Build history of the part. All positions in model axes, mm. Give positions to 0.01 mm unless a question says otherwise; leave off trailing zeros. Order: outer loops, then holes, each group sorted by start corner. A loop starts at its lowest first (then second) coordinate and runs counter-clockwise, first axis right, second up. Notation, with made-up numbers: (42, -31.5) - (60, -31.5) arc R13 cw to (60, -9.5) - close; hole circle Ø6 at (4, -28). An arc over 180 degrees is marked (long way). Use a Markdown table: item, result.
from build123d import *

# Parameters (mm, degrees)
SKETCH1_W           = 63.5
SKETCH1_H           = 88.9
SKETCH1_R           = 3.429
BOSS_EXTRUDE1_DEPTH = 6
FILLET1_R           = 10.16
SKETCH2_R           = 2.54
CUT_EXTRUDE1_DEPTH  = 110.414167273


with BuildPart() as part:
    # Sketch1 → Boss-Extrude1 (new body)
    with BuildSketch(Plane(origin=(0, 0, 0), x_dir=(1, 0, 0), z_dir=(0, 1, 0))):
        with Locations((31.75, 44.45)):
            Rectangle(SKETCH1_W, SKETCH1_H)
        with Locations(Location((17.78, 73.025, 0), (0, 0, 270))):
            Circle(SKETCH1_R, mode=Mode.SUBTRACT)
        with Locations(Location((45.72, 15.875, 0), (0, 0, 270))):
            Circle(SKETCH1_R, mode=Mode.SUBTRACT)
        with Locations(Location((17.78, 15.875, 0), (0, 0, 90))):
            Circle(SKETCH1_R, mode=Mode.SUBTRACT)
        with Locations(Location((45.72, 73.025, 0), (0, 0, 90))):
            Circle(SKETCH1_R, mode=Mode.SUBTRACT)
    extrude(amount=BOSS_EXTRUDE1_DEPTH)

    # Fillet1
    fillet1_edges = [part.edges().sort_by_distance(p)[0] for p in [
        (0, 3, -88.9),
        (63.5, 3, -88.9),
        (63.5, 3, 0),
        (0, 3, 0),
    ]]
    fillet(fillet1_edges, radius=FILLET1_R)

    # Sketch2 → Cut-Extrude1 (cut, through all)
    with BuildSketch(Plane(origin=(0, 6, 0), x_dir=(1, 0, 0), z_dir=(0, 1, 0))):
        with Locations(Location((6.35, 31.75, 0), (0, 0, 270))):
            Circle(SKETCH2_R)
        with Locations(Location((6.35, 44.45, 0), (0, 0, 270))):
            Circle(SKETCH2_R)
        with Locations(Location((6.35, 57.15, 0), (0, 0, 270))):
            Circle(SKETCH2_R)
        with Locations(Location((19.05, 57.15, 0), (0, 0, 270))):
            Circle(SKETCH2_R)
        with Locations(Location((19.05, 44.45, 0), (0, 0, 270))):
            Circle(SKETCH2_R)
        with Locations(Location((19.05, 31.75, 0), (0, 0, 270))):
            Circle(SKETCH2_R)
        with Locations(Location((31.75, 31.75, 0), (0, 0, 270))):
            Circle(SKETCH2_R)
        with Locations(Location((31.75, 44.45, 0), (0, 0, 270))):
            Circle(SKETCH2_R)
        with Locations(Location((31.75, 57.15, 0), (0, 0, 270))):
            Circle(SKETCH2_R)
        with Locations(Location((44.45, 57.15, 0), (0, 0, 270))):
            Circle(SKETCH2_R)
        with Locations(Location((44.45, 44.45, 0), (0, 0, 270))):
            Circle(SKETCH2_R)
        with Locations(Location((57.15, 44.45, 0), (0, 0, 270))):
            Circle(SKETCH2_R)
        with Locations(Location((57.15, 31.75, 0), (0, 0, 270))):
            Circle(SKETCH2_R)
        with Locations(Location((44.45, 31.75, 0), (0, 0, 270))):
            Circle(SKETCH2_R)
        with Locations(Location((57.15, 57.15, 0), (0, 0, 270))):
            Circle(SKETCH2_R)
    extrude(amount=-CUT_EXTRUDE1_DEPTH, mode=Mode.SUBTRACT)


solid = part.part
1) Two-plate mould, pull along X, no slides. Class faces 1 (the flat face through (63.5, 3, -44)), 2 (the cylindrical face through (17.63, 2.96, -12.45)), 3 (the cylindrical face through (2.897, 3.042, -3.055)): +X half, -X half, draft (parallel to the pull), parting line (faces both ways), or undercut.
Computed:
| item | result |
|---|---|
| face 1 | +X half |
| face 2 | undercut |
| face 3 | -X half |
2) Slice it at B-B (y = 2.6). State how many separate pieces and enclosed holes the cut face has, and give its area (3 significant figures).
Computed:
| item | result |
|---|---|
| separate pieces | 1 |
| enclosed holes | 19 |
| area | 5,100 mm² |
3) Slice it at C-C (z = -31.75). Write the cut outline in (x, y).
Computed:
| item | result |
|---|---|
| outline | (0, 0) - (3.81, 0) - (3.81, 6) - (0, 6) - close; (8.89, 0) - (16.51, 0) - (16.51, 6) - (8.89, 6) - close; (21.59, 0) - (29.21, 0) - (29.21, 6) - (21.59, 6) - close; (34.29, 0) - (41.91, 0) - (41.91, 6) - (34.29, 6) - close; (46.99, 0) - (54.61, 0) - (54.61, 6) - (46.99, 6) - close; (59.69, 0) - (63.5, 0) - (63.5, 6) - (59.69, 6) - close |
4) Slice it at A-A (x = 31.75). Write the cut outline in (y, z).
Computed:
| item | result |
|---|---|
| outline | (0, -88.9) - (6, -88.9) - (6, -59.69) - (0, -59.69) - close; (0, -54.61) - (6, -54.61) - (6, -46.99) - (0, -46.99) - close; (0, -41.91) - (6, -41.91) - (6, -34.29) - (0, -34.29) - close; (0, -29.21) - (6, -29.21) - (6, 0) - (0, 0) - close |
5) Slice it at D-D (x = 45.72). Write the cut outline in (y, z).
Computed:
| item | result |
|---|---|
| outline | (0, -88.9) - (6, -88.9) - (6, -76.45) - (0, -76.45) - close; (0, -69.6) - (6, -69.6) - (6, -59.35) - (0, -59.35) - close; (0, -54.95) - (6, -54.95) - (6, -46.65) - (0, -46.65) - close; (0, -42.25) - (6, -42.25) - (6, -33.95) - (0, -33.95) - close; (0, -29.55) - (6, -29.55) - (6, -19.3) - (0, -19.3) - close; (0, -12.45) - (6, -12.45) - (6, 0) - (0, 0) - close |
6) Wall check: line 1 (X direction, y = 4.45, z = -16); line 2 (X direction, y = 1.6, z = -57.15); line 3 (Z direction, x = 55, y = 4.5). Give the ranges that are in metal, low to high. Write a range as from..to.
Computed:
| item | result |
|---|---|
| line 1 | x = 0..14.35, 21.21..42.29, 49.15..63.5 |
| line 2 | x = 0..3.81, 8.89..16.51, 21.59..29.21, 34.29..41.91, 46.99..54.61, 59.69..63.5 |
| line 3 | z = -88.76..-58.5, -55.8..-45.8, -43.1..-33.1, -30.4..-0.14 |
